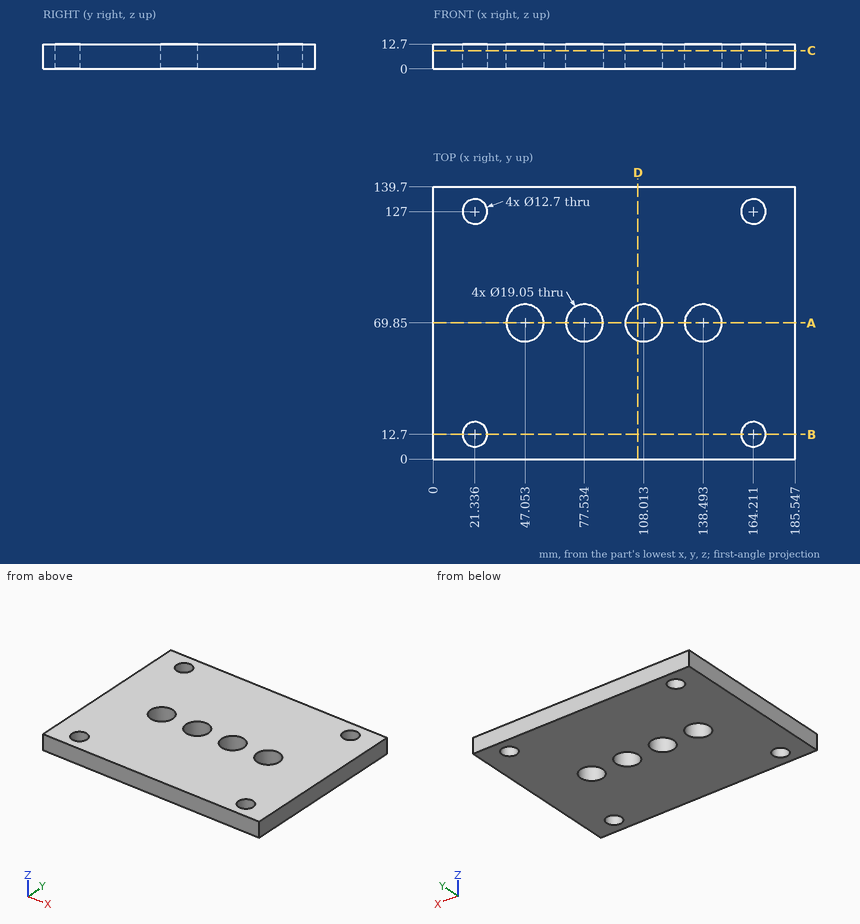
Drawing for the job (mm, zero at the part's lowest x, y, z). Give positions to 0.01 mm unless a question says otherwise; leave off trailing zeros. Write each loop counter-clockwise with the first axis right and the second up, starting at its lowest first coordinate (ties: lowest second). Pieces come first, ordered by that corner, then holes. Notation, with made-up numbers: (15.5, 46) - (19.5, 46) arc R19 cw to (19.5, 55) - close; hole circle Ø7 at (80.5, -39). An arc over 180 degrees is marked (long way). Answer as CSV lines item,"result".
Q1. Drill centre lines: line 1 (Y direction, x = 108, z = 9.5) (1 decimal); line 2 (Y direction, x = 161, z = 8.75); line 3 (Y direction, x = 20.5, z = 5.5) (1 decimal). Where is each one in solid material? Low to high. Write a range as from..to.
Result set:
line 1,"0..60.3, 79.4..139.7"
line 2,"0..7.22, 18.18..121.52, 132.48..139.7"
line 3,"0..6.4, 19..120.7, 133.3..139.7"
Q2. Flat gauge pin, fed straight in: pin 1 Ø7.5 at (x, y) = (21.336, 12.7) entering from +Z. Where does the tip first touch, or does it go through?
Result set:
pin 1,"through"
Q3. Band-saw the part on B-B (y = 12.7). Give the cut face in (x, z) (1 decimal), and give its area (3 significant figures).
Result set:
outline,"(0, 0) - (15, 0) - (15, 12.7) - (0, 12.7) - close; (27.7, 0) - (157.9, 0) - (157.9, 12.7) - (27.7, 12.7) - close; (170.6, 0) - (185.5, 0) - (185.5, 12.7) - (170.6, 12.7) - close"
area,"2,030 mm²"
Q4. Band-saw the part on D-D (x = 105). Give the cut face in (y, z) (1 decimal), and give its area (3 significant figures).
Result set:
outline,"(0, 0) - (60.8, 0) - (60.8, 12.7) - (0, 12.7) - close; (78.9, 0) - (139.7, 0) - (139.7, 12.7) - (78.9, 12.7) - close"
area,"1,540 mm²"
Q5. Band-saw the part on A-A (y = 69.85). Give the cut face in (x, z).
Result set:
outline,"(0, 0) - (37.53, 0) - (37.53, 12.7) - (0, 12.7) - close; (56.58, 0) - (68.01, 0) - (68.01, 12.7) - (56.58, 12.7) - close; (87.06, 0) - (98.49, 0) - (98.49, 12.7) - (87.06, 12.7) - close; (117.54, 0) - (128.97, 0) - (128.97, 12.7) - (117.54, 12.7) - close; (148.02, 0) - (185.55, 0) - (185.55, 12.7) - (148.02, 12.7) - close"
Q6. Band-saw the part on C-C (z = 9.25). State how many separate pieces and enclosed holes the cut face has, and give its area (3 significant figures).
Result set:
separate pieces,"1"
enclosed holes,"8"
area,"24,300 mm²"
